Check sheet for the modelled part. Datum: model origin and axes. Units: mm. A direction names the side the tool comes from. Round coordinates to 2 decimals unless told otherwise and drop trailing zeros. Write each loop counter-clockwise with the first axis right and the second up, starting at its lowest first coordinate (ties: lowest second). Pieces come first, ordered by that corner, then holes. Notation, with made-up numbers: M 1.25,70 L 15.25,70 A5 ccw 15.25,76 Z; hole C -13,72 d10. An arc over 180 degrees is marked long. One line per item, written item: value.
Autodesk Inventor part; units mm, degrees
ref_plane "YZ Plane" through (0, 0, 0) normal (1, 0, 0) x (0, 1, 0)
ref_plane "XZ Plane" through (0, 0, 0) normal (0, 1, 0) x (-1, 0, 0)
ref_plane "XY Plane" through (0, 0, 0) normal (0, 0, 1) x (1, 0, 0)
sketch "Sketch1" plane through (0, 0, 0) normal (0, 1, 0) x (-1, 0, 0)
  line L0 (0, 0) -> (-50, 0)
  line L1 (-50, 0) -> (-50, -100)
  line L2 (-50, -100) -> (0, -100)
  line L3 (0, -100) -> (0, 0)
  dimension "d0" = 50
  dimension "d1" = 100
extrude "Extrusion1" add sketch "Sketch1" along normal blind 65
sketch "Sketch2" plane through (50, 0, 0) normal (1, 0, 0) x (0, 0, -1)
  line L0 (0, 0) -> (100, 0)
  line L1 (50, 0) -> (50, 25)
  circle A0 centre (50, 25) radius 12
  line L2 (0, 65) -> (100, 65)
  line L3 (50, 65) -> (50, 25)
  dimension "d5" = 24
  dimension "d15" = 40
  dimension "d16" = 40
extrude "Extrusion2" cut sketch "Sketch2" against normal blind 65
sketch "Sketch3" plane through (0, 0, -100) normal (-1, 0, 0) x (0, 0, 1)
  circle A0 centre (50, 25) radius 12
  line L0 (0, 0) -> (100, 0)
  line L1 (62.5625, 0) -> (38, 0)
  circle A1 centre (50, 25) radius 12
  line L2 (0, 0) -> (100, 0)
  line L3 (100, 0) -> (100, 65)
  line L4 (0, 65) -> (100, 65)
  line L5 (0, 0) -> (0, 65)
  line L6 (62, 25) -> (62, 0)
  line L7 (38, 25) -> (38, 0)
  line L8 (100, 0) -> (0, 0)
extrude "Extrusion3" cut sketch "Sketch3" against normal blind 65 contours L6 L0 L7 A0
sketch "Sketch4" plane through (0, 0, 0) normal (0, -1, 0) x (1, 0, 0)
  line L0 (0, -100) -> (0, 0)
  line L1 (0, -100) -> (35, -100)
  line L2 (35, -100) -> (35, -70)
  line L3 (35, -70) -> (0, -70)
  line L4 (0, -70) -> (0, -100)
  line L5 (0, 0) -> (50, 0)
  line L6 (0, 0) -> (35, 0)
  line L7 (35, 0) -> (35, -30)
  line L8 (35, -30) -> (0, -30)
  line L9 (0, -30) -> (0, 0)
  dimension "d10" = 35
  dimension "d11" = 30
  dimension "d12" = 30
extrude "Extrusion4" cut sketch "Sketch4" against normal blind 50
sketch "Sketch5" plane through (0, 65, -100) normal (-1, 0, 0) x (0, 0, 1)
  line L0 (0, -15) -> (30, -15)
  line L1 (30, -15) -> (30, -65)
  line L2 (30, -65) -> (38, -65)
  line L3 (38, -65) -> (38, -40)
  arc A0 (62, -40) -> (38, -40) centre (50, -40) ccw
  line L4 (62, -40) -> (62, -65)
  line L5 (62, -65) -> (70, -65)
  line L6 (70, -65) -> (70, -15)
  line L7 (70, -15) -> (100, -15)
  line L8 (100, -15) -> (100, 0)
  line L9 (0, 0) -> (100, 0)
  line L10 (0, -15) -> (0, 0)
  line L11 (70, -15) -> (30, -15)
  point P0 (100, -65)
extrude "Extrusion5" cut sketch "Sketch5" against normal blind 4 contours L11 L6 L5 L4 A0 L3 L2 L1
sketch "Sketch6" plane through (35, 0, -70) normal (0, 0, -1) x (-1, 0, 0)
  circle A0 centre (16, 15) radius 5
  line L0 (31, 0) -> (31, 50)
  line L1 (31, 0) -> (0, 0)
  point P0 (35, 0)
  dimension "d19" = 10
  dimension "d20" = 15
  dimension "d21" = 15
extrude "Extrusion6" cut sketch "Sketch6" against normal through all
chamfer "Chamfer1" distance 15 angle 45 2 edges at (4, 0, -34) (4, 0, -66)
fillet "Fillet1" radius 15 4 edges at (42.5, 0, 0) (42.5, 0, -100) (0, 57.5, -100) (0, 57.5, 0)
sketch "Sketch7" plane through (0, 50, 0) normal (0, -1, 0) x (1, 0, 0)
  circle A0 centre (15, -85) radius 6
  circle A1 centre (15, -15) radius 6
  line L0 (0, -85) -> (0, -15)
  line L1 (15, 0) -> (35, 0)
  line L2 (35, -100) -> (15, -100)
  point P0 (0, 0)
  dimension "d28" = 12
  dimension "d29" = 12
  dimension "d30" = 15
  dimension "d31" = 15
  dimension "d32" = 15
  dimension "d33" = 15
extrude "Extrusion7" cut sketch "Sketch7" against normal through all
properties part number "Block4" material "Brass, Soft Yellow"
Q1. Sectioned sample at D-D on z = -50. Enter the section's corners in (x, y).
Completed:
outline: M 0,50 L 4,50 L 4,37 L 50,37 L 50,65 L 0,65 Z
Q2. Sectioned sample at C-C on x = 38.5. Enter the section's corners in (y, z), and give its area (3 significant figures).
Completed:
outline: M 0,-85 A15 ccw 15,-100 L 65,-100 L 65,0 L 15,0 A15 ccw 0,-15 L 0,-38 L 25,-38 A12 cw 25,-62 L 0,-62 Z
area: 5,580 mm^2
Q3. Draft check along X on faces 1 (the flat face through (38, 0, -29)), 2 (the cylindrical face through (20.08, 10.12, -66.06)), 3 (the flat face through (0, 57, -50)). Enter one of: pulls with the +X half, pulls with the -X half, needs draft (parallel to the pull), parting line crosses it, or undercut.
Completed:
face 1: needs draft
face 2: undercut
face 3: pulls with the -X half
Q4. Scan lines: line 1 (Z direction, x = 15, y = 56); line 2 (Z direction, x = 39, y = 25.5); line 3 (Y direction, x = 19, z = -65). Record each from-to range of solid material in increasing order. Write a range as [from, to].
Completed:
line 1: [-100, -91], [-79, -21], [-9, 0]
line 2: [-100, -61.99], [-38.01, 0]
line 3: [0, 10], [20, 65]
Q5. Sectioned sample at A-A on z = -66.5. Enter the section's corners in (x, y).
Completed:
outline: M 0,50 L 4,50 L 4,15 L 19,0 L 50,0 L 50,65 L 0,65 Z; hole C 19,15 d10
Q6. Access from +Z, -Z, +X, -X, +Y, -Y to the whole of each face (thin tool, end or side, straight path). Record for faces 4 (the flat face through (35, 25, -85)), 5 (the cylindrical face through (4.51, 57.6, -95.72)), 6 (the flat face through (4, 37, -55)), 7 (the flat face through (32, 13, -38)), 8 (the flat face through (35, 25, -15)).
Completed:
face 4: -Z, -X, -Y
face 5: -Z, -X, +Y, -Y
face 6: +Z, -Z, -X, -Y
face 7: +X, -X, -Y
face 8: +Z, -X, -Y
Q7. Depth check by flat-ended pin: P1, Ø8, axis at x = 23.5, y = 41, coming from the -Z side; P2, Ø12.5, axis at x = 23.5, y = 12, coming from the +Z side; P3, Ø5, axis at x = 5.5, y = 49.5, coming from the -Z side. Enter the tip coordinate at first touch or a pass-through.
Completed:
P1: z = -70
P2: z = -30
P3: z = -98.24
Q8. Sectioned sample at B-B on y = 59.5. Enter the section's corners in (x, z).
Completed:
outline: M 0,-85 A15 ccw 15,-100 L 50,-100 L 50,0 L 15,0 A15 ccw 0,-15 Z; hole C 15,-85 d12; hole C 15,-15 d12
